The listing builds one solid part. Answer for the finished solid, in the listing's coordinates (mm). Coordinates: 2 decimals unless noted, no trailing zeros. Write each loop counter-clockwise with the first axis right and the second up, starting at its lowest first coordinate (ties: lowest second). Pieces come first, ordered by that corner, then holes. Notation, with made-up numbers: M 22.25,-9 L 57.25,-9 A13 ccw 57.25,16 Z; hole C 17.25,31 d2. An arc over 180 degrees is marked long. Answer as CSV lines item,"result".
Autodesk Inventor part; units mm, degrees
ref_plane "YZ Plane" through (0, 0, 0) normal (1, 0, 0) x (0, 1, 0)
ref_plane "XZ Plane" through (0, 0, 0) normal (0, 1, 0) x (-1, 0, 0)
ref_plane "XY Plane" through (0, 0, 0) normal (0, 0, 1) x (1, 0, 0)
sketch "Sketch1" plane through (0, 0, 0) normal (0, 1, 0) x (-1, 0, 0)
  line L0 (0, 0) -> (12, 0)
  line L1 (12, 0) -> (12, -35)
  line L2 (12, -35) -> (0, -35)
  line L3 (0, -35) -> (0, 0)
  dimension "d0" = 12
  dimension "d1" = 35
extrude "Extrusion1" add sketch "Sketch1" along normal blind 100
sketch "Sketch2" plane through (0, 0, 0) normal (1, 0, 0) x (0, 0, -1)
  circle A0 centre (10, 90) radius 3
  line L0 (0, 0) -> (0, 100)
  line L1 (0, 100) -> (35, 100)
  circle A1 centre (25, 90) radius 3
  circle A2 centre (10, 70) radius 3
  circle A3 centre (25, 70) radius 3
  circle A4 centre (7.5, 10) radius 3
  line L2 (0, 0) -> (35, 0)
  circle A5 centre (27.5, 10) radius 3
  circle A6 centre (7.5, 30) radius 3
  circle A7 centre (27.5, 30) radius 3
  dimension "d4" = 6
  dimension "d5" = 10
  dimension "d6" = 10
  dimension "d9" = 15
  dimension "d12" = 20
  dimension "d15" = 6
  dimension "d16" = 10
  dimension "d17" = 7.5
  dimension "d20" = 20
  dimension "d23" = 20
extrude "Extrusion2" cut sketch "Sketch2" against normal through all
fillet "Fillet1" radius 6 4 edges at (-6, 0, 0) (-6, 0, -35) (-6, 100, 0) (-6, 100, -35)
fillet "Fillet2" radius 3 16 edges at (0, 98.2426, -33.2426) (0, 100, -17.5) (0, 98.2426, -1.7574) (0, 50, 0) (0, 1.7574, -1.7574) (0, 0, -17.5) (0, 1.7574, -33.2426) (0, 50, -35) (-12, 98.2426, -33.2426) (-12, 100, -17.5) (-12, 98.2426, -1.7574) (-12, 50, 0) (-12, 1.7574, -1.7574) (-12, 0, -17.5) (-12, 1.7574, -33.2426) (-12, 50, -35)
properties part number "EboxTslotMountV2"
Q1. Find section A-A (y = 70). Give the vertices of the cut face in (x, z).
Output:
outline,"M -12,-32 A3 ccw -9,-35 L -3,-35 A3 ccw 0,-32 L 0,-28 L -12,-28 Z; M -12,-22 L 0,-22 L 0,-13 L -12,-13 Z; M -12,-7 L 0,-7 L 0,-3 A3 ccw -3,0 L -9,0 A3 ccw -12,-3 Z"
Q2. Find section D-D (y = 92). Give the vertices of the cut face in (x, z).
Output:
outline,"M -12,-32 A3 ccw -9,-35 L -3,-35 A3 ccw 0,-32 L 0,-27.24 L -12,-27.24 Z; M -12,-22.76 L 0,-22.76 L 0,-12.24 L -12,-12.24 Z; M -12,-7.76 L 0,-7.76 L 0,-3 A3 ccw -3,0 L -9,0 A3 ccw -12,-3 Z"
Q3. The mould has two halves that part along Y. Classify faces 1 (the cylindrical face through (-11.14, 50.62, -0.9)), 2 (the cylindrical face through (-5.92, 67.07, -9.35)), 3 (the cylindrical face through (-5.958, 98.196, -33.289)): pulls with the +Y half, pulls with the -Y half, needs draft (parallel to the pull), parting line crosses it, or undercut.
Output:
face 1,"needs draft"
face 2,"undercut"
face 3,"pulls with the +Y half"
Q4. Flat-ended cylindrical pins translate along their axes: pin 1 Ø1.5 at (x, y) = (-10.5, 51.5) entering from +Z; pin 2 Ø1 at (x, y) = (-10.5, 76) entering from -Z. Find the tip coordinate at first contact, or state that the pin passes through.
Output:
pin 1,"z = -0.1"
pin 2,"z = -34.83"
Q5. Straight lines are drawn through the part: line 1 (Y direction, x = -9, z = -7.5); line 2 (Y direction, x = -8.25, z = -10); line 3 (Z direction, x = -8, y = 28). For each, find the intervals that lie inside material, in ascending order.
Output:
line 1,"0 to 7, 13 to 27, 33 to 68.34, 71.66 to 88.34, 91.66 to 100"
line 2,"0 to 8.34, 11.66 to 28.34, 31.66 to 67, 73 to 87, 93 to 100"
line 3,"-35 to -29.74, -25.26 to -9.74, -5.26 to 0"
Q6. Find section C-C (y = 49). Give the vertices of the cut face in (x, z).
Output:
outline,"M -12,-32 A3 ccw -9,-35 L -3,-35 A3 ccw 0,-32 L 0,-3 A3 ccw -3,0 L -9,0 A3 ccw -12,-3 Z"
Q7. Find section B-B (x = -6). Count the separate pieces of the cut face and the enclosed holes in it, and give its area (3 significant figures).
Output:
separate pieces,"1"
enclosed holes,"8"
area,"3,240 mm2"
